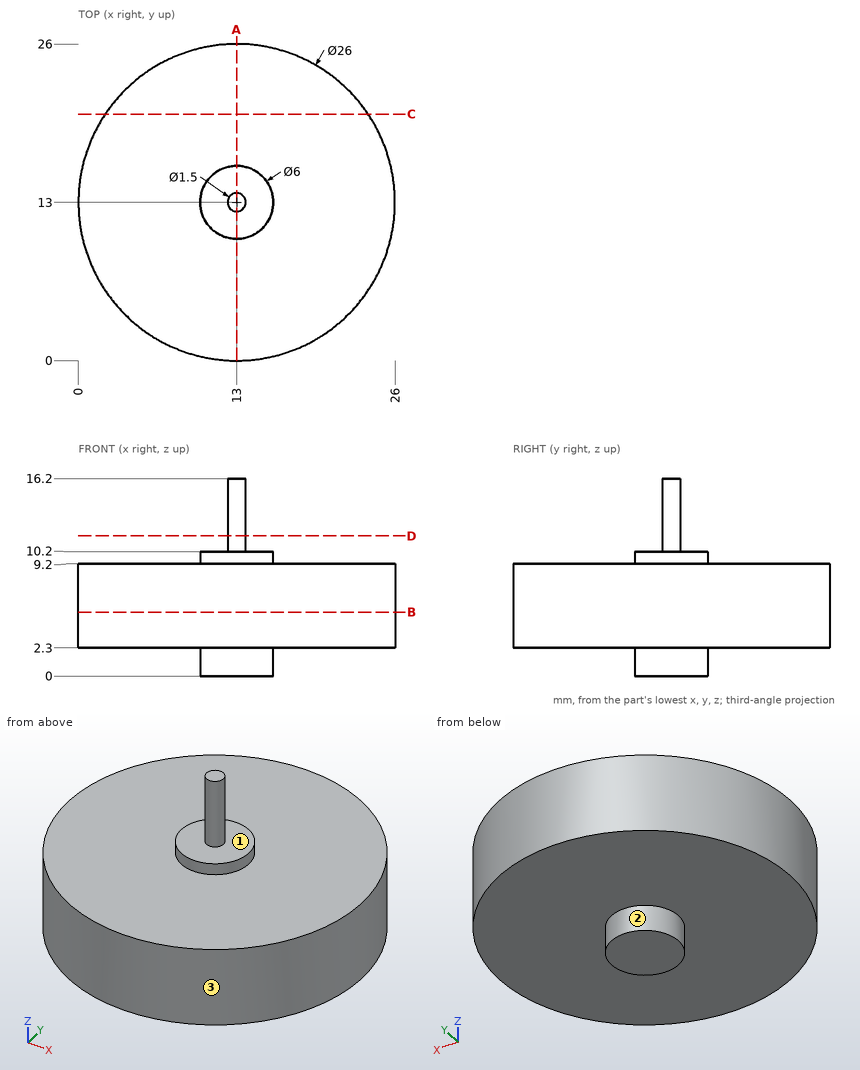
Source: three-view drawing plus pictorial views. Frame: mm from the lowest corner of the part. A direction names the side the tool comes from. Round coordinates to 2 decimals unless told otherwise and drop trailing zeros. Loops run counter-clockwise (first coordinate to the right, second up) from the corner with the lowest first, then second, coordinate; pieces in that order, holes last.
Item 1: Line query: L1, parallel to Z at x = 20, y = 5.5; L2, parallel to X at y = 14.75, z = 3; L3, parallel to X at y = 15.5, z = 7. Output: solid intervals per line, ascending.
Checked values:
L1: z = 2.3 to 9.2
L2: x = 0.12 to 25.88
L3: x = 0.24 to 25.76
Item 2: Section C-C, the plane y = 20.25. Output: boundary loops of the cut face in (x, z).
Checked values:
outline: (2.21, 2.3) - (23.79, 2.3) - (23.79, 9.2) - (2.21, 9.2) - close
Item 3: Reachability of the marked faces 1, 2 and 3 from +Z, -Z, +X, -X, +Y, -Y: full face, straight path, thin tool, end or side. Return the list, or none.
Checked values:
face 1: +Z
face 2: -Z
face 3: +Z, -Z
Item 4: Section A-A, the plane x = 13. Output: boundary loops of the cut face in (y, z), plus the area to 3 significant figures.
Checked values:
outline: (0, 2.3) - (10, 2.3) - (10, 0) - (16, 0) - (16, 2.3) - (26, 2.3) - (26, 9.2) - (16, 9.2) - (16, 10.2) - (13.75, 10.2) - (13.75, 16.2) - (12.25, 16.2) - (12.25, 10.2) - (10, 10.2) - (10, 9.2) - (0, 9.2) - close
area: 208 mm2
Item 5: Section B-B, the plane z = 5.25. Output: boundary loops of the cut face in (x, y), plus the area to 3 significant figures.
Checked values:
outline: circle Ø26 at (13, 13)
area: 531 mm2
Item 6: Contact query for flat-ended pins moving along their axis: P1, Ø5, axis at x = 18, y = 11, coming from the +Z side; P2, Ø3, axis at y = 16.5, z = 14, coming from the +X side; P3, Ø8, axis at x = 4, z = 2.5, coming from the +Y side; P4, Ø1, axis at x = 22, y = 8, coming from the +Z side. Output: stop coordinate, or through.
Checked values:
P1: stops at z = 10.2
P2: passes through
P3: stops at y = 25
P4: stops at z = 9.2
Item 7: Section D-D, the plane z = 11.5. Output: boundary loops of the cut face in (x, y), plus the area to 3 significant figures.
Checked values:
outline: circle Ø1.5 at (13, 13)
area: 1.77 mm2
